```python
from build123d import *

# Parameters (mm, degrees)
SKETCH1_W           = 400
SKETCH1_H           = 400
BOSS_EXTRUDE1_DEPTH = 700
CUT_EXTRUDE1_DEPTH  = 700
SKETCH4_W           = 200
SKETCH4_H           = 200
CUT_EXTRUDE2_DEPTH  = 700
CUT_EXTRUDE3_DEPTH  = 300
FILLET1_R           = 200
SKETCH6_R           = 50
CUT_EXTRUDE4_DEPTH  = 300
FILLET2_R           = 200
SKETCH7_R           = 50
CUT_EXTRUDE5_DEPTH  = 228
SKETCH8_R           = 50
CUT_EXTRUDE6_DEPTH  = 708


with BuildPart() as part:
    # Sketch1 → Boss-Extrude1 (new body)
    with BuildSketch(Plane(origin=(0, 0, 0), x_dir=(0, 0, -1), z_dir=(1, 0, 0))):
        with Locations((200, 200)):
            Rectangle(SKETCH1_W, SKETCH1_H)
    extrude(amount=-BOSS_EXTRUDE1_DEPTH)

    # Sketch2 → Cut-Extrude1 (cut)
    with BuildSketch(Plane(origin=(0, 0, 0), x_dir=(0, 0, -1), z_dir=(1, 0, 0))):
        Polygon((0, 400), (0, 100), (200, 400), align=None)
    extrude(amount=-CUT_EXTRUDE1_DEPTH, mode=Mode.SUBTRACT)

    # Sketch4 → Cut-Extrude2 (cut)
    with BuildSketch(Plane(origin=(0, 0, -400), x_dir=(-1, 0, 0), z_dir=(0, 0, -1))):
        with Locations((500, 300)):
            Rectangle(SKETCH4_W, SKETCH4_H)
    extrude(amount=-CUT_EXTRUDE2_DEPTH, mode=Mode.SUBTRACT)

    # Sketch5 → Cut-Extrude3 (cut)
    with BuildSketch(Plane(origin=(0, 0, 0), x_dir=(0, 0, -1), z_dir=(1, 0, 0))):
        Polygon((0, 100), (300, 100), (300, 300), (400, 300), (400, 400), (200, 400), align=None)
    extrude(amount=-CUT_EXTRUDE3_DEPTH, mode=Mode.SUBTRACT)

    # Fillet1
    fillet1_edges = [part.edges().sort_by_distance(p)[0] for p in [
        (0, 300, -350),
    ]]
    fillet(fillet1_edges, radius=FILLET1_R)

    # Sketch6 → Cut-Extrude4 (cut)
    with BuildSketch(Plane(origin=(0, 100, 0), x_dir=(1, 0, 0), z_dir=(0, 1, 0))):
        with Locations(Location((-150, 150, 0), (0, 0, 270))):
            Circle(SKETCH6_R)
    extrude(amount=-CUT_EXTRUDE4_DEPTH, mode=Mode.SUBTRACT)

    # Fillet2
    fillet2_edges = [part.edges().sort_by_distance(p)[0] for p in [
        (0, 50, 0),
    ]]
    fillet(fillet2_edges, radius=FILLET2_R)

    # Sketch7 → Cut-Extrude5 (cut)
    with BuildSketch(Plane.XY.offset(-300)):
        with Locations((-150, 180)):
            Circle(SKETCH7_R)
    extrude(amount=-CUT_EXTRUDE5_DEPTH, mode=Mode.SUBTRACT)

    # Sketch8 → Cut-Extrude6 (cut)
    with BuildSketch(Plane.ZY.offset(700)):
        with Locations(Location((-250, 300, 0), (0, 0, 180))):
            Circle(SKETCH8_R)
    extrude(amount=-CUT_EXTRUDE6_DEPTH, mode=Mode.SUBTRACT)


solid = part.part
```
Verification items for the finished model (mm, model axes). A direction names the side the tool comes from. Give positions to 0.01 mm unless a question says otherwise; leave off trailing zeros. Order: outer loops, then holes, each group sorted by start corner. A loop starts at its lowest first (then second) coordinate and runs counter-clockwise, first axis right, second up. Notation, with made-up numbers: (64.25, -21.75) - (107.25, -21.75) arc R15 cw to (107.25, 6.25) - close; hole circle Ø9 at (-22, 52.25). An arc over 180 degrees is marked (long way). Answer as CSV lines item,"result". Start each with the question number.
Item 1: Mould release check, pull along X, two halves, no side actions. Record for faces 4 (the face through (-300, 252, -197)), 5 (the face through (-190, 150, -349)), 6 (the face through (-181, 221, -300)): released by +X, released by -X, zero draft, split by the parting line, or undercut.
Item 2: Gauge pin test, flat ends, axial feed: pin 1 (1.5 mm diameter, centred on x = -279.5, y = 242.5, fed in from +Z); pin 2 (1 mm diameter, centred on x = -437.5, z = -280.5, fed in from +Y); pin 3 (1.5 mm diameter, centred on x = -490, y = 148, fed in from +Z); pin 4 (10 mm diameter, centred on x = -118.5, z = -239, fed in from -Y). Record the tip position at first contact, or that the pin passes through.
Item 3: Section check D-D, the plane y = 76.5. Record the boundary of the cut face in (x, z), plus the area to 3 significant figures.
Item 4: Section check B-B, the plane z = -318. Record the boundary of the cut face in (x, y).
Item 5: Access from +Z, -Z, +X, -X, +Y, -Y to the whole of each face (thin tool, end or side, straight path). Record for faces 1 (the face through (-600, 254, -273)), 2 (the face through (-249, 300, -349)), 3 (the face through (-349, 400, -299)).
Item 6: Section check C-C, the plane x = -184.5. Record the boundary of the cut face in (y, z).
Item 7: Section check A-A, the plane z = -250. Record the boundary of the cut face in (x, y), plus the area to 3 significant figures.
Item 8: Material ranges on L1, parallel to Y at x = -361.5, z = -250; L2, parallel to X at y = 369.5, z = -290; L3, parallel to Y at x = -61, z = -258, recorded low to high.
Filled in:
1,face 4,"released by +X"
1,face 5,"undercut"
1,face 6,"zero draft"
2,pin 1,"z = -300"
2,pin 2,"y = 200"
2,pin 3,"z = -31.5"
2,pin 4,"y = 0"
3,outline,"(-700, -400) - (0, -400) - (0, -200) arc R200 ccw to (-200, 0) - (-700, 0) - close; hole circle Ø100 at (-150, -150)"
3,area,"264,000 mm^2"
4,outline,"(-700, 0) - (0, 0) - (0, 100) arc R200 ccw to (-200, 300) - (-300, 300) - (-300, 400) - (-400, 400) - (-400, 200) - (-600, 200) - (-600, 400) - (-700, 400) - close; hole circle Ø100 at (-150, 180)"
5,face 1,"+Z, -Z, +Y"
5,face 2,"+Z, -Z, +X, +Y"
5,face 3,"+Z, -Z, +X, -X, +Y"
6,outline,"(0, -400) - (143.81, -400) - (143.81, -300) - (100, -300) - (100, -186.19) - (0, -186.19) - close; (0, -113.81) - (100, -113.81) - (100, -0.6) - (0, -0.6) - close; (216.19, -400) - (299.4, -400) - (299.4, -300) - (216.19, -300) - close"
7,outline,"(-700, 0) - (0, 0) - (0, 100) - (-300, 100) - (-300, 250) - (-400, 250) - (-400, 200) - (-600, 200) - (-600, 250) - (-700, 250) - close; (-700, 350) - (-600, 350) - (-600, 400) - (-700, 400) - close; (-400, 350) - (-300, 350) - (-300, 400) - (-400, 400) - close"
7,area,"130,000 mm^2"
8,L1,"0 to 250, 350 to 400"
8,L2,"-700 to -600, -400 to -300"
8,L3,"0 to 100"
